Can you work these out from the model? Positions are in its coordinate system, mm. Face numbers are marked on the shaded views. A direction names the side the tool comes from. Coordinates: 2 decimals unless noted, no trailing zeros. Loops run counter-clockwise (first coordinate to the right, second up) from the corner with the lowest first, then second, coordinate; pieces in that order, holes last.
```python
from build123d import *

# Parameters (mm, degrees)
SALIENTE_EXTRUIR1_DEPTH    = 2
CROQUIS2_W                 = 13.9
CROQUIS2_H                 = 20
SALIENTE_EXTRUIR2_DEPTH    = 24.5
SALIENTE_EXTRUIR3_DEPTH    = 22.5
CORTAR_EXTRUIR1_DEPTH      = 27
CORTAR_EXTRUIR1_DEPTH_BACK = 65.5
CROQUIS4_R                 = 1.599999999
REDONDEO1_R                = 3
REDONDEO2_R                = 5
CORTAR_EXTRUIR3_START      = 5
CORTAR_EXTRUIR3_DEPTH      = 3
CORTAR_EXTRUIR4_START      = -2
CORTAR_EXTRUIR4_DEPTH      = 3
CORTAR_EXTRUIR5_START      = -1
CORTAR_EXTRUIR5_DEPTH      = 3
CORTAR_EXTRUIR6_START      = 3
CORTAR_EXTRUIR6_DEPTH      = 3
SALIENTE_EXTRUIR5_START    = 2
SALIENTE_EXTRUIR5_DEPTH    = 2
CORTAR_EXTRUIR8_START      = -22.5
CROQUIS16_W                = 2.6
CROQUIS16_H                = 6.725582711
CROQUIS16_H_2              = 9.694654401
CORTAR_EXTRUIR8_DEPTH      = 22.5
CORTAR_EXTRUIR7_DEPTH      = 3
CORTAR_EXTRUIR7_DEPTH_BACK = 2
CROQUIS13_W                = 10
CROQUIS13_H                = 6.5
REDONDEO6_R                = 2
REDONDEO7_R                = 2
CROQUIS5_R                 = 1.25
CORTAR_EXTRUIR2_DEPTH      = 83.5


# Read off the part's stored shape, not the designer's step: Saliente-Extruir3
with BuildPart() as part:
    # Croquis1 → Saliente-Extruir1 (new body)
    with BuildSketch(Plane(origin=(0, 0, 0), x_dir=(1, 0, 0), z_dir=(0, 1, 0))):
        with BuildLine():
            Line((-31.5, -9.464532567), (31.5, -9.464532567))
            Line((31.5, -9.464532567), (31.5, 7.964532567))
            ThreePointArc((31.5, 7.964532567), (31.060660172, 9.025192739), (30, 9.464532567))
            Line((30, 9.464532567), (28.160101256, 9.464532567))
            ThreePointArc((28.160101256, 9.464532567), (27.099441084, 9.903872396), (26.660101256, 10.964532567))
            Line((26.660101256, 10.964532567), (26.660101256, 14.266885585))
            ThreePointArc((26.660101256, 14.266885585), (20.802236879, 28.409021208), (6.660101256, 34.266885585))
            Line((6.660101256, 34.266885585), (-6.660101256, 34.266885585))
            ThreePointArc((-6.660101256, 34.266885585), (-20.802236879, 28.409021208), (-26.660101256, 14.266885585))
            Line((-26.660101256, 14.266885585), (-26.660101256, 10.964532567))
            ThreePointArc((-26.660101256, 10.964532567), (-27.099441084, 9.903872396), (-28.160101256, 9.464532567))
            Line((-28.160101256, 9.464532567), (-30, 9.464532567))
            ThreePointArc((-30, 9.464532567), (-31.060660172, 9.025192739), (-31.5, 7.964532567))
            Line((-31.5, 7.964532567), (-31.5, -9.464532567))
        make_face()
    extrude(amount=SALIENTE_EXTRUIR1_DEPTH)

    # Croquis2 → Saliente-Extruir2 (add)
    with BuildSketch(Plane(origin=(0, 0, 0), x_dir=(1, 0, 0), z_dir=(0, 1, 0))):
        Rectangle(CROQUIS2_W, CROQUIS2_H)
    extrude(amount=SALIENTE_EXTRUIR2_DEPTH)

    # Saliente-Extruir3 outline → Saliente-Extruir3 (add)
    with BuildSketch(Plane(origin=(0, 2, 0), x_dir=(1, 0, 0), z_dir=(0, 1, 0))):
        with BuildLine():
            Line((-31.5, 7.964532567), (-31.5, -0.75))
            Line((-31.5, -0.75), (-25.6, -0.75))
            Line((-25.6, -0.75), (-25.6, 10.285420177))
            Line((-25.6, 10.285420177), (-26.822638598, 10.285420177))
            ThreePointArc((-26.822638598, 10.285420177), (-27.375457574, 9.686121721), (-28.160101256, 9.464532567))
            Line((-28.160101256, 9.464532567), (-30, 9.464532567))
            ThreePointArc((-30, 9.464532567), (-31.060660172, 9.025192739), (-31.5, 7.964532567))
        make_face()
        with BuildLine():
            Line((31.5, -0.75), (31.5, 7.964532567))
            ThreePointArc((31.5, 7.964532567), (31.060660172, 9.025192739), (30, 9.464532567))
            Line((30, 9.464532567), (28.160101256, 9.464532567))
            ThreePointArc((28.160101256, 9.464532567), (27.375457574, 9.686121721), (26.822638598, 10.285420177))
            Line((26.822638598, 10.285420177), (25.6, 10.285420177))
            Line((25.6, 10.285420177), (25.6, -0.75))
            Line((25.6, -0.75), (31.5, -0.75))
        make_face()
    extrude(amount=SALIENTE_EXTRUIR3_DEPTH)

    # Croquis4 → Cortar-Extruir1 (cut, two sides: drawn at the far end of the back side and taken through both)
    with BuildSketch(Plane.ZY.offset(25.5).offset(-CORTAR_EXTRUIR1_DEPTH_BACK)):
        with Locations((-6.002353017, 4.3)):
            Circle(CROQUIS4_R)
        with Locations((-6.002353017, 22.4)):
            Circle(CROQUIS4_R)
    extrude(amount=CORTAR_EXTRUIR1_DEPTH + CORTAR_EXTRUIR1_DEPTH_BACK, mode=Mode.SUBTRACT)

    # Redondeo1
    redondeo1_edges = [part.edges().sort_by_distance(p)[0] for p in [
        (0, 24.5, 10),
        (-28.55, 2, 0.75),
        (28.55, 2, 0.75),
    ]]
    fillet(redondeo1_edges, radius=REDONDEO1_R)

    # Redondeo2
    redondeo2_edges = [part.edges().sort_by_distance(p)[0] for p in [
        (0, 2, -10),
    ]]
    fillet(redondeo2_edges, radius=REDONDEO2_R)

    # Croquis8 → Cortar-Extruir3 (cut)
    with BuildSketch(Plane(origin=(0, 0, 0), x_dir=(0, 0, -1), z_dir=(1, 0, 0)).offset(CORTAR_EXTRUIR3_START)):
        Polygon((2.752353017, 22.4), (4.377353017, 19.585417438), (7.627353017, 19.585417438), (9.252353017, 22.4), (7.627353017, 25.214582562), (4.377353017, 25.214582562), align=None)
    extrude(amount=-CORTAR_EXTRUIR3_DEPTH, mode=Mode.SUBTRACT)

    # Croquis9 → Cortar-Extruir4 (cut)
    with BuildSketch(Plane(origin=(0, 0, 0), x_dir=(0, 0, -1), z_dir=(1, 0, 0)).offset(CORTAR_EXTRUIR4_START)):
        Polygon((2.752353017, 22.4), (4.377353017, 19.585417438), (7.627353017, 19.585417438), (9.252353017, 22.4), (7.627353017, 25.214582562), (4.377353017, 25.214582562), align=None)
    extrude(amount=-CORTAR_EXTRUIR4_DEPTH, mode=Mode.SUBTRACT)

    # Croquis10 → Cortar-Extruir5 (cut)
    with BuildSketch(Plane(origin=(0, 0, 0), x_dir=(0, 0, -1), z_dir=(1, 0, 0)).offset(CORTAR_EXTRUIR5_START)):
        Polygon((6.002353017, 7.55), (3.187770455, 5.925), (3.187770455, 2.675), (6.002353017, 1.05), (8.816935579, 2.675), (8.816935579, 5.925), align=None)
    extrude(amount=-CORTAR_EXTRUIR5_DEPTH, mode=Mode.SUBTRACT)

    # Croquis11 → Cortar-Extruir6 (cut)
    with BuildSketch(Plane(origin=(0, 0, 0), x_dir=(0, 0, -1), z_dir=(1, 0, 0)).offset(CORTAR_EXTRUIR6_START)):
        Polygon((2.752353017, 4.3), (4.377353017, 1.485417438), (7.627353017, 1.485417438), (9.252353017, 4.3), (7.627353017, 7.114582562), (4.377353017, 7.114582562), align=None)
    extrude(amount=-CORTAR_EXTRUIR6_DEPTH, mode=Mode.SUBTRACT)

    # Croquis15 → Saliente-Extruir5 (add)
    with BuildSketch(Plane.XZ.offset(SALIENTE_EXTRUIR5_START)):
        with BuildLine():
            Line((-31.5, 9.464532567), (31.5, 9.464532567))
            Line((31.5, 9.464532567), (31.5, -7.489095092))
            ThreePointArc((31.5, -7.489095092), (30.914213562, -8.903308654), (29.5, -9.489095092))
            Line((29.5, -9.489095092), (28.660101256, -9.489095092))
            ThreePointArc((28.660101256, -9.489095092), (27.245887693, -10.074881529), (26.660101256, -11.489095092))
            Line((26.660101256, -11.489095092), (26.660101256, -14.266885585))
            ThreePointArc((26.660101256, -14.266885585), (20.802236879, -28.409021208), (6.660101256, -34.266885585))
            Line((6.660101256, -34.266885585), (1.137553535, -34.266885585))
            Line((1.137553535, -34.266885585), (-1.137553535, -34.266885585))
            Line((-1.137553535, -34.266885585), (-6.660101256, -34.266885585))
            ThreePointArc((-6.660101256, -34.266885585), (-20.802236879, -28.409021208), (-26.660101256, -14.266885585))
            Line((-26.660101256, -14.266885585), (-26.660101256, -11.489095092))
            ThreePointArc((-26.660101256, -11.489095092), (-27.245887693, -10.074881529), (-28.660101256, -9.489095092))
            Line((-28.660101256, -9.489095092), (-29.5, -9.489095092))
            ThreePointArc((-29.5, -9.489095092), (-30.914213562, -8.903308654), (-31.5, -7.489095092))
            Line((-31.5, -7.489095092), (-31.5, 9.464532567))
        make_face()
    extrude(amount=-SALIENTE_EXTRUIR5_DEPTH)

    # Croquis16 → Cortar-Extruir8 (cut)
    with BuildSketch(Plane(origin=(0, 24.5, 0), x_dir=(1, 0, 0), z_dir=(0, 1, 0)).offset(CORTAR_EXTRUIR8_START)):
        with Locations((5.65, -3.637208644)):
            Rectangle(CROQUIS16_W, CROQUIS16_H)
        with Locations((5.65, -11.847327201)):
            Rectangle(CROQUIS16_W, CROQUIS16_H_2)
        with Locations((-5.65, -11.847327201)):
            Rectangle(CROQUIS16_W, CROQUIS16_H_2)
        with Locations((-5.65, -3.637208644)):
            Rectangle(CROQUIS16_W, CROQUIS16_H)
    extrude(amount=CORTAR_EXTRUIR8_DEPTH, mode=Mode.SUBTRACT)

    # Croquis13 → Cortar-Extruir7 (cut, two sides: drawn at the far end of the back side and taken through both)
    with BuildSketch(Plane.XZ.offset(-CORTAR_EXTRUIR7_DEPTH_BACK)):
        with Locations((0, -6.002353017)):
            Rectangle(CROQUIS13_W, CROQUIS13_H)
    extrude(amount=CORTAR_EXTRUIR7_DEPTH + CORTAR_EXTRUIR7_DEPTH_BACK, mode=Mode.SUBTRACT)

    # Redondeo6
    redondeo6_edges = [part.edges().sort_by_distance(p)[0] for p in [
        (-31.5, -2, 0.987718738),
        (-30.914213562, -2, -8.903308654),
        (-29.080050628, -2, -9.489095092),
        (-27.245887693, -2, -10.074881529),
        (-26.660101256, -2, -12.877990338),
        (-20.802236879, -2, -28.409021208),
        (0, -2, -34.266885585),
        (20.802236879, -2, -28.409021208),
        (26.660101256, -2, -12.877990338),
        (27.245887693, -2, -10.074881529),
        (29.080050628, -2, -9.489095092),
        (30.914213562, -2, -8.903308654),
        (31.5, -2, 0.987718738),
    ]]
    fillet(redondeo6_edges, radius=REDONDEO6_R - 0.0001)  # a hair under: the kernel refuses the full size

    # Redondeo7
    redondeo7_edges = [part.edges().sort_by_distance(p)[0] for p in [
        (31.5, 0.99995, 9.464532567),
        (-31.5, 0.99995, 9.464532567),
        (0, -2, 9.464532567),
        (30.914242852, -1.414242852, 9.464532567),
        (-30.914242852, -1.414242852, 9.464532567),
    ]]
    fillet(redondeo7_edges, radius=REDONDEO7_R - 0.0001)  # a hair under: the kernel refuses the full size

    # Croquis5 → Cortar-Extruir2 (cut)
    with BuildSketch(Plane(origin=(0, 24.5, 0), x_dir=(1, 0, 0), z_dir=(0, 1, 0))):
        with Locations(Location((0, 1.798301608, 0), (0, 0, 270))):
            Circle(CROQUIS5_R)
        with Locations(Location((0, -6.026932469, 0), (0, 0, 308.880755469))):
            Circle(CROQUIS5_R)
        with Locations(Location((-28.55, 1.798301608, 0), (0, 0, 270))):
            Circle(CROQUIS5_R)
        with Locations(Location((28.55, 1.798301608, 0), (0, 0, 270))):
            Circle(CROQUIS5_R)
    extrude(amount=-CORTAR_EXTRUIR2_DEPTH, mode=Mode.SUBTRACT)


solid = part.part
```
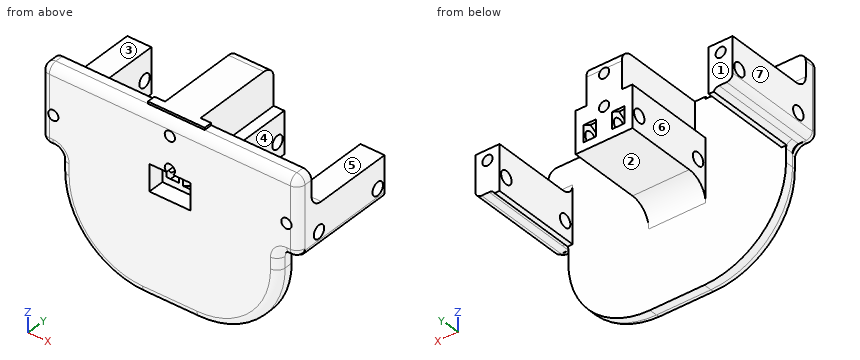
(1) If we mould it in two halves opening along X, with no side actions, what happens to the marked faces 5, 6 and 7? For each: released by +X, released by -X, zero draft, split by the parting line, or undercut.
Check values:
face 5: zero draft
face 6: undercut
face 7: released by -X
(2) Which directions (+Z, -Z, +X, -X, +Y, -Y) give clear straight access to the entire face, cutting with the end or side of a thin tool? Please do the marked faces 1, 2, 3 and 4.
Check values:
face 1: +Z, -Z, +X, -X, +Y
face 2: -Z, +Y
face 3: +Z, -X, +Y
face 4: +Z, -Z, +Y
(3) I want a section at A-A on y = 17. Write out the boundary of the cut face in (x, z).
Check values:
outline: (-31.5, -7.96) arc R1.5 ccw to (-30, -9.46) - (-28.16, -9.46) arc R1.5 cw to (-26.82, -10.29) - (-25.6, -10.29) - (-25.6, 0.75) - (-31.5, 0.75) - close; (-6.95, -10) - (6.95, -10) - (6.95, 0.27) - (4.35, 0.27) - (4.35, 10) - (-4.35, 10) - (-4.35, 0.27) - (-6.95, 0.27) - close; (25.6, -10.29) - (26.82, -10.29) arc R1.5 cw to (28.16, -9.46) - (30, -9.46) arc R1.5 ccw to (31.5, -7.96) - (31.5, 0.75) - (25.6, 0.75) - close; hole circle Ø2.5 at (-28.55, -1.8); hole circle Ø2.5 at (0, -1.8); hole circle Ø2.5 at (0, 6.03); hole circle Ø2.5 at (28.55, -1.8)
(4) If I drill on probe 1 along Z at (x, y) = (-28.6, 22.4); probe 2 along Z at (x, y) = (0, 9); probe 3 along X at (y, z) = (20.5, -5), over which ranges is the centre line in solid material (lowest first)?
Check values:
probe 1: z = -9.46 to -7.6, -4.4 to -3.05, -0.55 to 0.75
probe 2: z = -10 to -3.05, -0.55 to 4.78, 7.28 to 10
probe 3: x = -31.5 to -25.6, -6.95 to -5, -2 to 2, 5 to 6.95, 25.6 to 31.5
(5) I'm going to push flat-ended pins straight in: pin 1 (3 mm diameter, centred on x = -28.55, z = -1.8, fed in from -Y); pin 2 (1.5 mm diameter, centred on x = 0, z = -1.8, fed in from +Y); pin 3 (2 mm diameter, centred on x = -9.5, z = -14, fed in from +Y); pin 4 (0.9 mm diameter, centred on x = -3, z = -6.5, fed in from +Y). Where does each tip first touch, or does it pass through?
Check values:
pin 1: stops at y = -2
pin 2: passes through
pin 3: stops at y = 2
pin 4: stops at y = 19.59
